CAD build for the part. Positions are in the model's coordinates, mm. Face numbers are marked on the shaded views. A direction names the side the tool comes from. Round coordinates to 2 decimals unless told otherwise and drop trailing zeros. Loops run counter-clockwise (first coordinate to the right, second up) from the corner with the lowest first, then second, coordinate; pieces in that order, holes last.
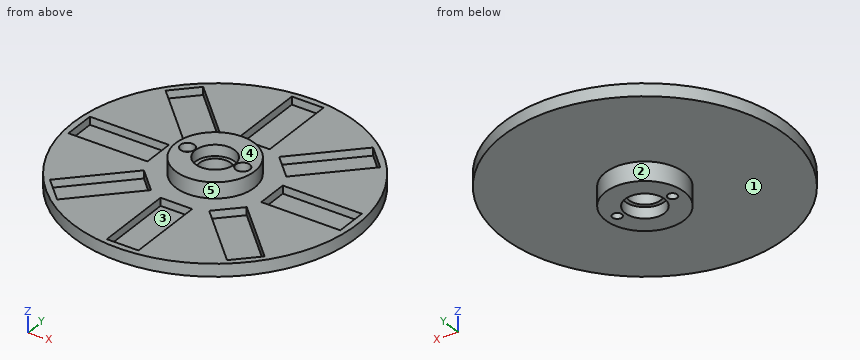
```python
from build123d import *

# Parameters (mm, degrees)
SKETCH_R             = 90
PAD_DEPTH            = 8
SKETCH001_W          = 20
SKETCH001_H          = 50
POCKET_DEPTH         = 5
SKETCH002_W          = 20
SKETCH002_H          = 50
POCKET001_DEPTH      = 5
SKETCH003_W          = 50
SKETCH003_H          = 20
POCKET002_DEPTH      = 5
SKETCH004_W          = 50
SKETCH004_H          = 20
POCKET003_DEPTH      = 5
POCKET004_DEPTH      = 5
POCKET005_DEPTH      = 5
POCKET006_DEPTH      = 5
POCKET007_DEPTH      = 5
SKETCH009_R          = 25
PAD001_DEPTH         = 20
PAD001_DEPTH_BACK    = 10
SKETCH010_R          = 10
HOLE_DEPTH           = 30.001
SKETCH011_R          = 12.5
POCKET008_DEPTH      = 7
SKETCH012_R          = 12.5
POCKET009_DEPTH      = 7
HOLE001_D            = 6
HOLE001_CBORE_D      = 9
HOLE001_CBORE_DEPTH  = 5.4
BODY_PLACEMENT_ANGLE = 180


with BuildPart() as part:
    # Sketch → Pad (new body)
    with BuildSketch(Plane.XY):
        Circle(SKETCH_R)
    extrude(amount=PAD_DEPTH)

    # Sketch001 → Pocket (cut)
    with BuildSketch(Plane.XY):
        with Locations((0, 61)):
            Rectangle(SKETCH001_W, SKETCH001_H)
    extrude(amount=POCKET_DEPTH, mode=Mode.SUBTRACT)

    # Sketch002 → Pocket001 (cut)
    with BuildSketch(Plane.XY):
        with Locations((0, -61)):
            Rectangle(SKETCH002_W, SKETCH002_H)
    extrude(amount=POCKET001_DEPTH, mode=Mode.SUBTRACT)

    # Sketch003 → Pocket002 (cut)
    with BuildSketch(Plane.XY):
        with Locations((61, 0)):
            Rectangle(SKETCH003_W, SKETCH003_H)
    extrude(amount=POCKET002_DEPTH, mode=Mode.SUBTRACT)

    # Sketch004 → Pocket003 (cut)
    with BuildSketch(Plane.XY):
        with Locations((-61, 0)):
            Rectangle(SKETCH004_W, SKETCH004_H)
    extrude(amount=POCKET003_DEPTH, mode=Mode.SUBTRACT)

    # Sketch005 → Pocket004 (cut)
    with BuildSketch(Plane.XY):
        Polygon((-67.882251, 53.740115), (-32.526912, 18.384776), (-18.384776, 32.526912), (-53.740115, 67.882251), align=None)
    extrude(amount=POCKET004_DEPTH, mode=Mode.SUBTRACT)

    # Sketch006 → Pocket005 (cut)
    with BuildSketch(Plane.XY):
        Polygon((18.384776, 32.526912), (32.526912, 18.384776), (67.882251, 53.740115), (53.740115, 67.882251), align=None)
    extrude(amount=POCKET005_DEPTH, mode=Mode.SUBTRACT)

    # Sketch007 → Pocket006 (cut)
    with BuildSketch(Plane.XY):
        Polygon((-67.882251, -53.740115), (-53.740115, -67.882251), (-18.384776, -32.526912), (-32.526912, -18.384776), align=None)
    extrude(amount=POCKET006_DEPTH, mode=Mode.SUBTRACT)

    # Sketch008 → Pocket007 (cut)
    with BuildSketch(Plane.XY):
        Polygon((18.384776, -32.526912), (32.526912, -18.384776), (67.882251, -53.740115), (53.740115, -67.882251), align=None)
    extrude(amount=POCKET007_DEPTH, mode=Mode.SUBTRACT)

    # Sketch009 → Pad001 (join, two sides)
    with BuildSketch(Plane.XY) as pad001_sk:
        Circle(SKETCH009_R)
    extrude(amount=PAD001_DEPTH)
    extrude(pad001_sk.sketch, amount=-PAD001_DEPTH_BACK)

    # Sketch010 (on Face42 of Pad001) → Hole (cut, through all)
    with BuildSketch(Plane(origin=(0, 0, -10), x_dir=(1, 0, 0), z_dir=(0, 0, -1))):
        Circle(SKETCH010_R)
    extrude(amount=-HOLE_DEPTH, mode=Mode.SUBTRACT)

    # Sketch011 (on Face42 of Hole) → Pocket008 (cut)
    with BuildSketch(Plane(origin=(0, 0, -10), x_dir=(1, 0, 0), z_dir=(0, 0, -1))):
        Circle(SKETCH011_R)
    extrude(amount=-POCKET008_DEPTH, mode=Mode.SUBTRACT)

    # Sketch012 (on Face47 of Pocket008) → Pocket009 (cut)
    with BuildSketch(Plane.XY.offset(20)):
        Circle(SKETCH012_R)
    extrude(amount=-POCKET009_DEPTH, mode=Mode.SUBTRACT)

    # Hole001 (through all)
    with Locations(Plane(origin=(0, 0, -10), x_dir=(1, 0, 0), z_dir=(0, 0, -1))):
        with Locations((0, 0), (17.5, 0), (-17.5, 0)):
            CounterBoreHole(HOLE001_D / 2, HOLE001_CBORE_D / 2, HOLE001_CBORE_DEPTH)


with BuildPart() as part_1:
    # Body placement: moved
    add(part.part.moved(Location((0, 0, 10))).rotate(Axis((0, 0, 10), (0, 1, 0)), BODY_PLACEMENT_ANGLE))


solid = part_1.part
```
Item 1: 3-axis set-ups, long thin cutter, end or side, ignore diameter. For the marked faces 4 and 5: which of +Z, -Z, +X, -X, +Y, -Y reach the whole face in a straight line?
Answers follow:
face 4: +Z, +X, -X, +Y, -Y
face 5: +Z
Item 2: Two-plate mould, pull along X, no slides. Class the marked faces 1, 2 and 3: released by +X, released by -X, zero draft, split by the parting line, or undercut.
Answers follow:
face 1: zero draft
face 2: split by the parting line
face 3: undercut
Item 3: Cut at C-C, the plane x = 48.5. Give the cut face in (y, z), plus the area to 3 significant figures.
Answers follow:
outline: (-75.81, 2) - (75.81, 2) - (75.81, 10) - (62.64, 10) - (62.64, 5) - (34.36, 5) - (34.36, 10) - (10, 10) - (10, 5) - (-10, 5) - (-10, 10) - (-34.36, 10) - (-34.36, 5) - (-62.64, 5) - (-62.64, 10) - (-75.81, 10) - close
area: 830 mm2
Item 4: Probe line 1 (Y direction, x = 6, z = 7); line 2 (Y direction, x = 0, z = -5); line 3 (Z direction, x = -62, y = 2). List the from-to ranges inside material, lowest first.
Answers follow:
line 1: y = -89.8 to -86, -36 to -8, 8 to 36, 86 to 89.8
line 2: y = -25 to -12.5, 12.5 to 25
line 3: z = 2 to 5
Item 5: Cut at D-D, the plane x = 28. Give the cut face in (y, z).
Answers follow:
outline: (-85.53, 2) - (85.53, 2) - (85.53, 10) - (42.14, 10) - (42.14, 5) - (22.91, 5) - (22.91, 10) - (-22.91, 10) - (-22.91, 5) - (-42.14, 5) - (-42.14, 10) - (-85.53, 10) - close
Item 6: Flat gauge pins, fed straight in: P1, Ø1.5, axis at y = -2, z = 6.5, coming from the +X side; P2, Ø12, axis at x = -39.5, z = -2.5, coming from the +Y side; P3, Ø10, axis at x = -3, y = 59, coming from the +Z side. Where does each tip first touch, or does it go through?
Answers follow:
P1: stops at x = 89.99
P2: stops at y = 82.69
P3: stops at z = 5
Item 7: Cut at B-B, the plane y = 0. State how many separate pieces and enclosed holes the cut face has, plus the area to 3 significant figures.
Answers follow:
separate pieces: 4
enclosed holes: 0
area: 978 mm2
